Work out the finished part from the listing and answer in its coordinate system (mm). Face numbers are marked on the shaded views. A direction names the side the tool comes from. Coordinates: 2 decimals unless noted, no trailing zeros. Order: outer loops, then holes, each group sorted by start corner. A loop starts at its lowest first (then second) coordinate and runs counter-clockwise, first axis right, second up. Notation, with made-up numbers: (44.5, 13.5) - (79.5, 13.5) arc R35 ccw to (79.5, 50.5) - close; hole circle Ø9 at (-28.75, 42.25). An arc over 180 degrees is marked (long way). Answer as a JSON object with one key per item and string values. Group by question number.
1) A tool of negligible diameter and unlimited length cuts with its end or side. For the marked faces 5 and 6, from which of +Z, -Z, +X, -X, +Y, -Y can it reach the whole face along a straight path? Write none if from no direction.
2) Section D-D (z = 28) is taken. Give the vertices of the cut face in (x, y).
3) Find the intervals of material crossed by line 1 along Y through (x, z) = (0, 6.25); line 2 along Y through (x, z) = (0, 17.75); line 3 along X through (y, z) = (0, 20), in increasing order.
4) Section A-A (y = 0) is taken. Give the vertices of the cut face in (x, z).
5) Section C-C (z = 10) is taken. Give the vertices of the cut face in (x, y) (1 decimal).
6) The mould has two halves that part along Y. Classify the marked faces 1, 2, 3 and 4: released by +Y, released by -Y, zero draft, split by the parting line, or undercut.
7) Section B-B (x = 0) is taken. Count the separate pieces of the cut face and the enclosed holes in it, plus the area to 3 significant figures.
8) Each of these flat-tipped pins is pushed along its axis until it touches: P1, Ø3, axis at y = 14, z = 10, coming from the +X side; P2, Ø3.5, axis at y = -17, z = 14.5, coming from the +X side; P3, Ø5, axis at x = -13.5, z = 17, coming from the +Y side; P4, Ø4, axis at x = -30.83, y = 30.83, coming from the +Z side. Where does it stop, or does it pass through?
from build123d import *

# Parameters (mm, degrees)
F0_W      = 76.2
F0_H      = 76.2
F0_R      = 3.175
F5_DEPTH  = 6.35
F1_R      = 13.7737792641
F6_DEPTH  = 25.4
F3_R      = 5.199817611
F7_DEPTH  = 25.4
F4_W      = 20.6375
F4_H      = 3.6285714286
F8_DEPTH  = 25.4
F2_R      = 32.3782922644
F2_W      = 20.6375
F2_H      = 3.6632169593
F9_DEPTH  = 25.4
F10_D     = 9.525
F11_R     = 16.0757593031
F11_R_2   = 13.7737792641
F11_R_3   = 1.27
F12_DEPTH = 6.35
F13_DEPTH = 29.21
F14_W     = 8.89
F14_H     = 8.3891552745
F15_DEPTH = 21.59


with BuildPart() as f5:
    # F0 (on Top) → F5 (new body)
    with BuildSketch(Plane.XY):
        Rectangle(F0_W, F0_H)
        with Locations((-30.7339914143, -30.8254174888)):
            Circle(F0_R, mode=Mode.SUBTRACT)
        with Locations((30.9182778001, -30.8254174888)):
            Circle(F0_R, mode=Mode.SUBTRACT)
        with Locations((-30.8268517256, 30.8268517256)):
            Circle(F0_R, mode=Mode.SUBTRACT)
        with Locations((31.2360748649, 30.8268517256)):
            Circle(F0_R, mode=Mode.SUBTRACT)
    extrude(amount=F5_DEPTH)

    # F1 (on face) → F6 (cut)
    with BuildSketch(Plane.XY):
        Circle(F1_R)
    extrude(amount=F6_DEPTH, mode=Mode.SUBTRACT)

    # F3 (on face) → F7 (cut)
    with BuildSketch(Plane.XY):
        with Locations((0, 22.2998782992)):
            Circle(F3_R)
    extrude(amount=F7_DEPTH, mode=Mode.SUBTRACT)

    # F4 (on face) → F8 (cut)
    with BuildSketch(Plane.XY):
        with Locations((0, -21.663627077)):
            Rectangle(F4_W, F4_H)
    extrude(amount=F8_DEPTH, mode=Mode.SUBTRACT)

    # F2 (on face) → F9 (join)
    with BuildSketch(Plane.XY):
        Circle(F2_R)
        with Locations((0.0286572114, -21.8153223838)):
            Rectangle(F2_W, F2_H, mode=Mode.SUBTRACT)
    extrude(amount=F9_DEPTH)

    # F10 (through all)
    with Locations(Plane(origin=(0, 0, 0), x_dir=(1, 0, 0), z_dir=(0, 0, -1))):
        with Locations((0, -22.2998782992)):
            Hole(F10_D / 2)

    # F11 (on face) → F12 (join)
    with BuildSketch(Plane.XY.offset(25.4)):
        Circle(F11_R)
        Circle(F11_R_2, mode=Mode.SUBTRACT)
        Circle(F11_R_2)
        Circle(F11_R_3, mode=Mode.SUBTRACT)
    extrude(amount=F12_DEPTH)

    # F1 (on face) → F13 (cut)
    with BuildSketch(Plane.XY):
        Circle(F1_R)
    extrude(amount=F13_DEPTH, mode=Mode.SUBTRACT)

    # F14 (on face) → F15 (cut)
    with BuildSketch(Plane.XY):
        with Locations((0, -16.7856216431)):
            Rectangle(F14_W, F14_H)
    extrude(amount=F15_DEPTH, mode=Mode.SUBTRACT)


solid = f5.part
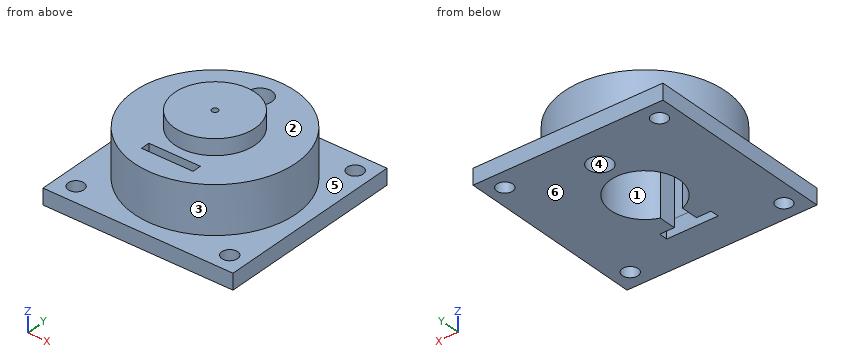
Report:
{
 "1": {"face 5": "+Z", "face 6": "-Z, +X, -X, +Y, -Y"},
 "2": {"outline": "circle Ø32.15 at (0, 0); hole circle Ø27.55 at (0, 0)"},
 "3": {"line 1": "y = -38.1 to -23.48, 13.77 to 17.54, 27.06 to 38.1", "line 2": "y = -32.38 to -23.65, 13.77 to 17.54, 27.06 to 32.38", "line 3": "x = -32.38 to -13.77, 13.77 to 32.38"},
 "4": {"outline": "(-38.1, 0) - (-13.77, 0) - (-13.77, 29.21) - (-1.27, 29.21) - (-1.27, 31.75) - (-16.08, 31.75) - (-16.08, 25.4) - (-32.38, 25.4) - (-32.38, 6.35) - (-38.1, 6.35) - close; (1.27, 29.21) - (13.77, 29.21) - (13.77, 0) - (38.1, 0) - (38.1, 6.35) - (32.38, 6.35) - (32.38, 25.4) - (16.08, 25.4) - (16.08, 31.75) - (1.27, 31.75) - close"},
 "5": {"outline": "circle Ø64.8 at (0, 0); hole (-10.3, -23.6) - (10.3, -23.6) - (10.3, -20) - (4.4, -20) - (4.4, -13) arc R13.8 ccw (long way) to (-4.4, -13) - (-4.4, -20) - (-10.3, -20) - close; hole circle Ø9.5 at (0, 22.3)"},
 "6": {"face 1": "undercut", "face 2": "zero draft", "face 3": "split by the parting line", "face 4": "undercut"},
 "7": {"separate pieces": "4", "enclosed holes": "0", "area": "643 mm²"},
 "8": {"P1": "stops at x = 29.87", "P2": "stops at x = 28.56", "P3": "stops at y = 30.45", "P4": "passes through"}
}
